from build123d import *

# Parameters (mm, degrees)
SKETCH_1_W          = 60
SKETCH_1_H          = 124
EXTRUDE_1_DEPTH     = 6
SKETCH_2_R          = 16.4
SKETCH_2_R_2        = 1.5
CUT_EXTRUDE_1_DEPTH = 7
SKETCH_4_R          = 2
CUT_EXTRUDE_2_DEPTH = 7
SKETCH_5_W          = 60
SKETCH_5_H          = 6
EXTRUDE_2_DEPTH     = 6
SKETCH_6_R          = 2
CUT_EXTRUDE_3_DEPTH = 7
SKETCH_7_R          = 5.65
SKETCH_7_R_2        = 2
SKETCH_7_W          = 10.5
SKETCH_7_H          = 20
EXTRUDE_3_DEPTH     = 6


with BuildPart() as part:
    # Эскиз1 → Бобышка-Вытянуть1 (new body)
    with BuildSketch(Plane.XY):
        Rectangle(SKETCH_1_W, SKETCH_1_H)
    extrude(amount=EXTRUDE_1_DEPTH)

    # Эскиз2 → Вырез-Вытянуть1 (cut, through all)
    with BuildSketch(Plane.XY.offset(6)):
        with Locations((0, 40.85)):
            Circle(SKETCH_2_R)
        with Locations((-15.5, 56.35)):
            Circle(SKETCH_2_R_2)
        with Locations((15.5, 56.35)):
            Circle(SKETCH_2_R_2)
        with Locations((15.5, 25.35)):
            Circle(SKETCH_2_R_2)
        with Locations((-15.5, 25.35)):
            Circle(SKETCH_2_R_2)
    extrude(amount=-CUT_EXTRUDE_1_DEPTH, mode=Mode.SUBTRACT)

    # Эскиз4 → Вырез-Вытянуть2 (cut, through all)
    with BuildSketch(Plane.XY.offset(6)):
        with Locations((-24.6, -55)):
            Circle(SKETCH_4_R)
        with Locations((0, -55)):
            Circle(SKETCH_4_R)
        with Locations((24.6, -55)):
            Circle(SKETCH_4_R)
    extrude(amount=-CUT_EXTRUDE_2_DEPTH, mode=Mode.SUBTRACT)

    # Эскиз5 → Бобышка-Вытянуть2 (add)
    with BuildSketch(Plane(origin=(0, 62, 0), x_dir=(1, 0, 0), z_dir=(0, 1, 0))):
        with Locations((0, -3)):
            Rectangle(SKETCH_5_W, SKETCH_5_H)
    extrude(amount=EXTRUDE_2_DEPTH)

    # Эскиз6 → Вырез-Вытянуть3 (cut, through all)
    with BuildSketch(Plane(origin=(0, 0, 0), x_dir=(-1, 0, 0), z_dir=(0, 0, -1))):
        with Locations((-25.75, 62.35)):
            Circle(SKETCH_6_R)
        with Locations((25.75, 62.35)):
            Circle(SKETCH_6_R)
        with Locations((25.75, 25.7)):
            Circle(SKETCH_6_R)
        with Locations((-25.75, 25.7)):
            Circle(SKETCH_6_R)
        with Locations((0, -18.3)):
            Circle(SKETCH_6_R)
    extrude(amount=-CUT_EXTRUDE_3_DEPTH, mode=Mode.SUBTRACT)

    # Эскиз7 → Бобышка-Вытянуть3 (add)
    with BuildSketch(Plane(origin=(0, 0, 0), x_dir=(-1, 0, 0), z_dir=(0, 0, -1))):
        with Locations((-25.75, 62.35)):
            Circle(SKETCH_7_R)
        with Locations((-25.75, 62.35)):
            Circle(SKETCH_7_R_2, mode=Mode.SUBTRACT)
        with Locations((25.75, 62.35)):
            Circle(SKETCH_7_R)
        with Locations((25.75, 62.35)):
            Circle(SKETCH_7_R_2, mode=Mode.SUBTRACT)
        with Locations((25.75, 25.7)):
            Circle(SKETCH_7_R)
        with Locations((25.75, 25.7)):
            Circle(SKETCH_7_R_2, mode=Mode.SUBTRACT)
        with Locations((-35.25, 28)):
            Rectangle(SKETCH_7_W, SKETCH_7_H)
    extrude(amount=-EXTRUDE_3_DEPTH)


solid = part.part
The model under review builds one solid part; all positions refer to its coordinate system, in mm. A direction names the side the tool comes from. Round coordinates to 2 decimals unless told otherwise and drop trailing zeros. Loops run counter-clockwise (first coordinate to the right, second up) from the corner with the lowest first, then second, coordinate; pieces in that order, holes last. Notation, with made-up numbers: M -38.5,-15.75 L 11.5,-15.75 A16 cw 11.5,10.25 Z; hole C 37,33 d9. An arc over 180 degrees is marked long. Answer as CSV lines item,"result". Start each with the question number.
Item 1: Mouldability with a two-part tool opening along X and no side actions: class faces 1 (the face through (35, 38, 3)), 2 (the face through (-17, 25.4, 3)), 3 (the face through (-31.4, 25.6, 3)), 4 (the face through (40.5, 28, 3)) as released by +X, released by -X, zero draft, split by the parting line, or undercut.
Item 2: For faces 5 (the face through (0, -53, 3)), 6 (the face through (-30, -21, 3)), 7 (the face through (4, 2, 0)), 8 (the face through (30, -23, 3)), 9 (the face through (30, 48, 3)), list the 3-axis set-ups (+Z, -Z, +X, -X, +Y, -Y) from which the entire face can be reached by the end or side of a thin tool; tool diameter is ignored.
Item 3: Consider section A-A (y = 40.85). Write out the cut boundary in (x, z), then the cut area to 3 significant figures.
Item 4: Consider section B-B (z = 1.3). State how many separate pieces and enclosed holes the cut face has, then the cut area to 3 significant figures.
Item 5: Wall thickness on line 1 (Y direction, x = 0, z = 2.7); line 2 (X direction, y = 56, z = 0.7); line 3 (X direction, y = 41, z = 2): over which ranges is each line inside the solid? List them lowest first. Write a range as [from, to].
Item 6: Consider section C-C (x = 25). Write out the cut boundary in (y, z).
Item 7: Consider section D-D (x = -4.5). Write out the cut boundary in (y, z).
Item 8: Insertion check: P1, Ø2, axis at y = -28, z = 2.5, coming from the -X side. The pin has a flat end and moves straight along its axis. Give the tip position at first contact, or say it passes through.
Answer:
1,face 1,"zero draft"
1,face 2,"undercut"
1,face 3,"released by -X"
1,face 4,"released by +X"
2,face 5,"+Z, -Z"
2,face 6,"+Z, -Z, -X, -Y"
2,face 7,"-Z, +X, -X, +Y, -Y"
2,face 8,"+Z, -Z, +X, -Y"
2,face 9,"+Z, -Z, +X"
3,outline,"M -30,0 L -16.4,0 L -16.4,6 L -30,6 Z; M 16.4,0 L 30,0 L 30,6 L 16.4,6 Z"
3,area,"163 mm^2"
4,separate pieces,"1"
4,enclosed holes,"13"
4,area,"7,060 mm^2"
5,line 1,"y = [-62, -57], [-53, -20.3], [-16.3, 24.45], [57.25, 68]"
5,line 2,"x = [-30, -16.96], [-14.04, -6.28], [6.28, 14.04], [16.96, 30]"
5,line 3,"x = [-30, -16.4], [16.4, 30]"
6,outline,"M -62,0 L -56.96,0 L -56.96,6 L -62,6 Z; M -53.04,0 L 23.85,0 L 23.85,6 L -53.04,6 Z; M 27.55,0 L 60.5,0 L 60.5,6 L 27.55,6 Z; M 64.2,0 L 68,0 L 68,6 L 64.2,6 Z"
7,outline,"M -62,0 L 25.08,0 L 25.08,6 L -62,6 Z; M 56.62,0 L 68,0 L 68,6 L 56.62,6 Z"
8,P1,"stops at x = -30"
